```python
from build123d import *

# Parameters (mm, degrees)
BOSS_EXTRUDE1_DEPTH     = 100
SHELL1_T                = -2
SKETCH4_W               = 14.567996804
SKETCH4_H               = 196
SKETCH4_W_2             = 15.490077846
BOSS_EXTRUDE2_DEPTH     = 1
CUT_EXTRUDE1_DEPTH      = 327.114830331
CUT_EXTRUDE1_DEPTH_BACK = 327.114830331
SKETCH5_R               = 8.25


with BuildPart() as part:
    # Sketch1 → Boss-Extrude1 (new, symmetric)
    with BuildSketch(Plane.XY):
        with BuildLine():
            Line((-157.3, 0), (-172.3, 0))
            Line((-172.3, 0), (-172.3, -3))
            Line((-172.3, -3), (172.3, -3))
            Line((172.3, -3), (172.3, 0))
            Line((172.3, 0), (157.3, 0))
            ThreePointArc((157.3, 0), (159.477998018, 71.943974663), (136.046041615, 140))
            Line((136.046041615, 140), (157.833839596, 152.259358023))
            Line((157.833839596, 152.259358023), (135.766995153, 191.477394389))
            Line((135.766995153, 191.477394389), (66.046041615, 152.247448714))
            ThreePointArc((66.046041615, 152.247448714), (-74.612286943, 118.644986984), (-157.3, 0))
        make_face()
    extrude(amount=BOSS_EXTRUDE1_DEPTH, both=True)

    # Shell1
    shell1_openings = [part.faces().sort_by_distance(p)[0] for p in [
        (146.800417374, 171.868376206, 0),
        (0, -3, 0),
    ]]
    offset(amount=SHELL1_T, openings=shell1_openings, kind=Kind.INTERSECTION)

    # Sketch4 → Boss-Extrude2 (add)
    with BuildSketch(Plane.XZ.offset(2)):
        with Locations((-163.016001598, 0)):
            Rectangle(SKETCH4_W, SKETCH4_H)
        with Locations((162.554961077, 0)):
            Rectangle(SKETCH4_W_2, SKETCH4_H)
    extrude(amount=BOSS_EXTRUDE2_DEPTH)

    # Sketch5 → Cut-Extrude1 (cut, two sides: drawn at the far end of the back side and taken through both)
    with BuildSketch(Plane.XY.offset(100).offset(-CUT_EXTRUDE1_DEPTH_BACK)):
        with Locations((0, 9.692663859)):
            Circle(SKETCH5_R)
    extrude(amount=CUT_EXTRUDE1_DEPTH + CUT_EXTRUDE1_DEPTH_BACK, mode=Mode.SUBTRACT)


solid = part.part
```
Model file for the job. Use its own axes, mm. A direction names the side the tool comes from. Give positions to 0.01 mm unless a question says otherwise; leave off trailing zeros. Write each loop counter-clockwise with the first axis right and the second up, starting at its lowest first coordinate (ties: lowest second). Pieces come first, ordered by that corner, then holes. Notation, with made-up numbers: M 67.25,16 L 112.25,16 A4 ccw 112.25,20 Z; hole C 44.5,74 d9. An arc over 180 degrees is marked long. Use a Markdown table: item, result.
1) Cut at C-C (y = 122). List the corners of the cut face in (x, z), and give its area (3 significant figures).
Responses:
| item | result |
|---|---|
| outline | M -69.53,-100 L 145.01,-100 L 145.01,100 L -69.53,100 Z; hole M -65.77,-98 L 142.83,-98 L 142.83,98 L -65.77,98 Z |
| area | 2,020 mm2 |
2) Tool access for faces 1 (the cylindrical face through (-1.79, 1.64, -99.01)), 2 (the cylindrical face through (157.69, 70.38, 1.37)), 3 (the flat face through (165, 0, 1)): list every direction of +Z, -Z, +X, -X, +Y, -Y with a clear straight run to the whole face (end or side of a thin tool).
Responses:
| item | result |
|---|---|
| face 1 | +Z, -Z |
| face 2 | none |
| face 3 | +Z, -Z, +X |
3) Drill centre lines: line 1 (Z direction, x = -82.5, y = 37.5); line 2 (X direction, y = 94.5, z = -79); line 3 (X direction, y = 135.5, z = 60.5). Where is each one in solid material? Low to high. Write a range as from..to.
Responses:
| item | result |
|---|---|
| line 1 | z = -100..-98, 98..100 |
| line 2 | x = -103.77..-100.93, 152.64..154.71 |
| line 3 | x = -44.75..-39.83, 136.24..138.5 |
4) Cut at A-A (z = 53.5). List the corners of the cut face in (x, y).
Responses:
| item | result |
|---|---|
| outline | M -172.3,-3 L -155.73,-3 L -155.73,-2 A201.2 cw 66.45,150.18 L 136.75,189.73 L 135.77,191.48 L 66.05,152.25 A203.2 ccw -157.3,0 L -172.3,0 Z; M 133.31,140.76 A198 cw 154.81,-2 L 154.81,-3 L 172.3,-3 L 172.3,0 L 157.3,0 A200 ccw 136.05,140 L 157.83,152.26 L 156.85,154 Z |
5) Pull direction X, two halves, no side cores. Call faces 4 (the cylindrical face through (159.628, 70.942, 1.4)), 5 (the flat face through (-165, 0, 1)), 6 (the cylindrical face through (-72.146, 117.898, 1.372)): +X half, -X half, draft (parallel to the pull), parting line (faces both ways), or undercut.
Responses:
| item | result |
|---|---|
| face 4 | +X half |
| face 5 | draft |
| face 6 | undercut |
6) Cut at B-B (x = 0). List the corners of the cut face in (y, z).
Responses:
| item | result |
|---|---|
| outline | M -3,-100 L 1.44,-100 L 1.44,-98 L -3,-98 Z; M -3,98 L 1.44,98 L 1.44,100 L -3,100 Z; M 17.94,-100 L 150,-100 L 150,100 L 17.94,100 L 17.94,98 L 147.96,98 L 147.96,-98 L 17.94,-98 Z |
7) Cut at D-D (y = 166.5). List the corners of the cut face in (x, z), and give its area (3 significant figures).
Responses:
| item | result |
|---|---|
| outline | M 91.38,-100 L 149.82,-100 L 149.82,-98 L 95.45,-98 L 95.45,98 L 149.82,98 L 149.82,100 L 91.38,100 Z |
| area | 1,030 mm2 |
8) Pin check, flat tips, straight feed: pin 1 (8 mm diameter, centred on x = 51, z = -45.5, fed in from -Y); pin 2 (12 mm diameter, centred on y = 131, z = -47.5, fed in from +X); pin 3 (4 mm diameter, centred on x = 106.5, z = -79, fed in from -Y). Stop position of each tip, or through.
Responses:
| item | result |
|---|---|
| pin 1 | stops at y = 151.37 |
| pin 2 | stops at x = 143.67 |
| pin 3 | stops at y = 171.59 |
